Geometry: final body of the model. Coordinates: model frame, mm. A direction names the side the tool comes from. Give positions to 0.01 mm unless a question says otherwise; leave off trailing zeros. Order: outer loops, then holes, each group sorted by start corner. A loop starts at its lowest first (then second) coordinate and runs counter-clockwise, first axis right, second up. Notation, with made-up numbers: (-28, 13.25) -> (-14, 13.25) arc R12 cw to (-14, 24.25) -> close; hole circle Ø7 at (31.25, -8.5). An arc over 180 degrees is marked (long way). Answer in a Markdown table with one row per item. Add a question column.
Q1. Pull-direction query (Z, two-part tool) for faces 1 (the face through (-36, 0, -22.225)), 2 (the face through (-0.484, 0.044, 1.378)), 3 (the face through (-36, 0, -3.175)), 4 (the face through (-27.305, 0, -31)); classes: +Z half, -Z half, draft (parallel to the pull), parting line (faces both ways), or undercut.
Q2. Cut plane B-B on z = 24. Return the cut outline in (x, y) (3 decimals).
Q3. Contact query for flat-ended pins moving along their axis: P1, Ø3, axis at x = -17, y = 0, coming from the -Z side; P2, Ø3, axis at x = -36.5, y = -0.5, coming from the +Z side (3 decimals); P3, Ø1.9, axis at y = 0.5, z = -31, coming from the +X side (3 decimals). Output: stop coordinate, or through.
Q4. Line query: line 1 along Z through (x, y) = (-6.35, 1); line 2 along Z through (x, y) = (23, -1.5); line 3 along X through (y, z) = (-0.5, 27). Output: solid intervals per line, ascending. Write a range as from..to.
Q5. Set-up query: faces 5 (the face through (-33.02, 0, -25)), 6 (the face through (20, 0, -27.94)), 7 (the face through (-18, 0, 27.94)). Return all of +Z, -Z, +X, -X, +Y, -Y with unobstructed straight access to the full face (end or side cutting, diameter ignored); none if empty.
Q6. Cut plane A-A on x = -6.35. Return the cut outline in (y, z) (3 decimals), and give its area (3 significant figures).
from build123d import *

# Parameters (mm, degrees)
F0_R     = 6.35
F1_DEPTH = 3.175


with BuildPart() as f1:
    # F0 (on Front) → F1 (new body, symmetric)
    with BuildSketch(Plane.XZ):
        Polygon((33.02, -27.94), (33.02, 27.94), (29.845, 27.94), (29.845, 34.29), (23.495, 34.29), (23.495, 27.94), (17.145, 27.94), (17.145, 34.29), (10.795, 34.29), (10.795, 27.94), (4.445, 27.94), (4.445, 34.29), (-1.905, 34.29), (-1.905, 27.94), (-8.255, 27.94), (-8.255, 34.29), (-14.605, 34.29), (-14.605, 27.94), (-20.955, 27.94), (-20.955, 34.29), (-27.305, 34.29), (-27.305, 27.94), (-33.02, 27.94), (-33.02, 22.225), (-39.37, 22.225), (-39.37, 15.875), (-33.02, 15.875), (-33.02, 9.525), (-39.37, 9.525), (-39.37, 3.175), (-33.02, 3.175), (-33.02, -3.175), (-39.37, -3.175), (-39.37, -9.475044), (-33.02, -9.475044), (-33.02, -9.525), (-33.02, -15.875), (-39.37, -15.875), (-39.37, -22.225), (-33.02, -22.225), (-33.02, -27.94), (-27.305, -27.94), (-27.305, -34.29), (-20.955, -34.29), (-20.955, -27.94), (-14.605, -27.94), (-14.605, -34.29), (-8.255, -34.29), (-8.255, -27.94), (-1.905, -27.94), (-1.905, -34.29), (4.445, -34.29), (4.445, -27.94), (10.795, -27.94), (10.795, -34.29), (17.145, -34.29), (17.145, -27.94), (23.495, -27.94), (23.495, -34.29), (29.845, -34.29), (29.845, -27.94), align=None)
        with Locations((-6.35, 3.81)):
            Circle(F0_R, mode=Mode.SUBTRACT)
    extrude(amount=F1_DEPTH, both=True)


solid = f1.part
Completed:
| question | item | result |
|---|---|---|
| 1 | face 1 | -Z half |
| 1 | face 2 | undercut |
| 1 | face 3 | undercut |
| 1 | face 4 | draft |
| 2 | outline | (-33.02, -3.175) -> (33.02, -3.175) -> (33.02, 3.175) -> (-33.02, 3.175) -> close |
| 3 | P1 | stops at z = -27.94 |
| 3 | P2 | stops at z = 22.225 |
| 3 | P3 | stops at x = 29.845 |
| 4 | line 1 | z = -27.94..-2.54, 10.16..27.94 |
| 4 | line 2 | z = -27.94..27.94 |
| 4 | line 3 | x = -33.02..33.02 |
| 5 | face 5 | -Z, -X, +Y, -Y |
| 5 | face 6 | -Z, +Y, -Y |
| 5 | face 7 | +Z, +Y, -Y |
| 6 | outline | (-3.175, -27.94) -> (3.175, -27.94) -> (3.175, -2.54) -> (-3.175, -2.54) -> close; (-3.175, 10.16) -> (3.175, 10.16) -> (3.175, 27.94) -> (-3.175, 27.94) -> close |
| 6 | area | 274 mm² |
